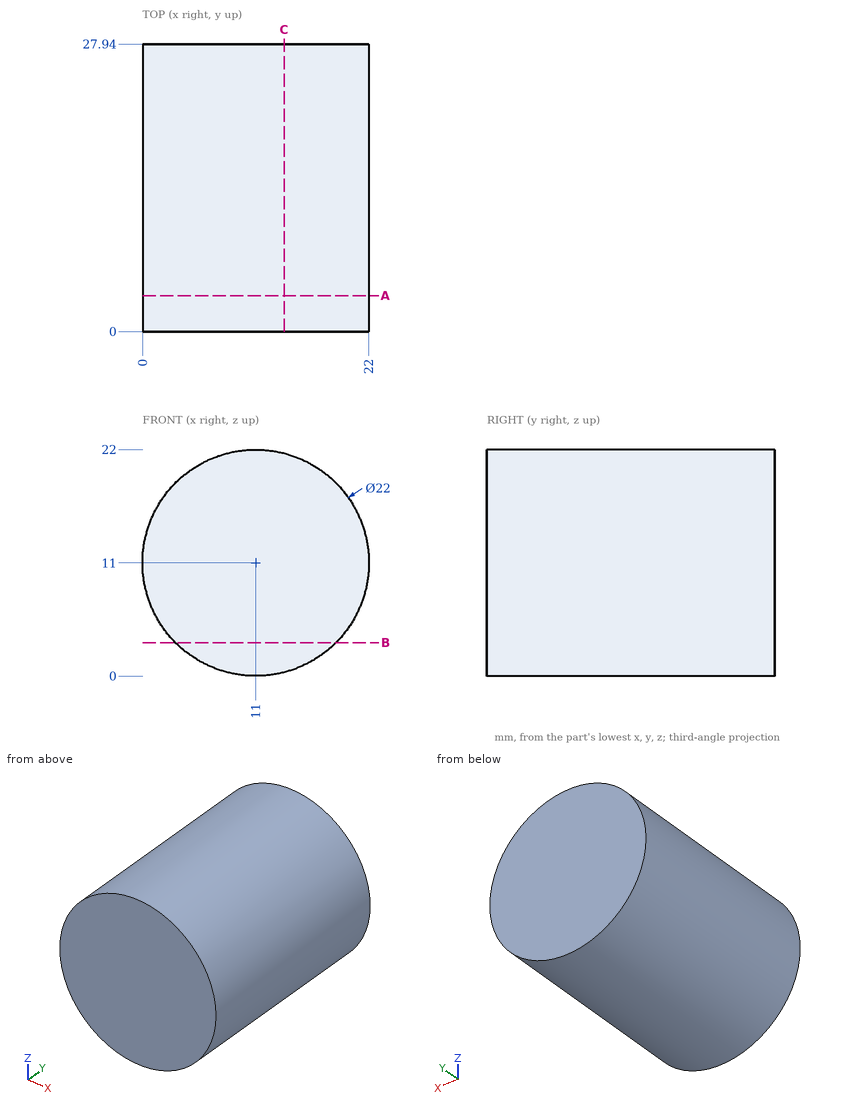
Geometry check sheet. Reference: drawing and pictorial views, mm from the part's lowest x, y, z. Give positions to 0.01 mm unless a question says otherwise; leave off trailing zeros. Order: outer loops, then holes, each group sorted by start corner. A loop starts at its lowest first (then second) coordinate and runs counter-clockwise, first axis right, second up. Notation, with made-up numbers: (-29.5, 74.25) -> (5.5, 74.25) arc R23 ccw to (5.5, 103.25) -> close; hole circle Ø1 at (71.5, 7). An arc over 180 degrees is marked (long way). Write each question's results on one line, items separated by ' | '. Start each with the question number.
(1) Gauge pin test, flat end, axial feed: P1, Ø8, axis at y = 13, z = 4.5, coming from the +X side. Record the tip position at first contact, or that the pin passes through.
(2) Sectioned sample at B-B (z = 3.25). Enter the section's corners in (x, y).
(3) Sectioned sample at A-A (y = 3.5). Enter the section's corners in (x, z), plus the area to 3 significant figures.
(4) Scan lines: line 1 (Z direction, x = 10.75, y = 21.25); line 2 (Z direction, x = 3.5, y = 11); line 3 (X direction, y = 26, z = 6.75). Record each from-to range of solid material in increasing order.
(5) Sectioned sample at C-C (x = 13.75). Enter the section's corners in (y, z), plus the area to 3 significant figures.
Answer below:
1) P1: x = 21.71
2) outline: (3.19, 0) -> (18.81, 0) -> (18.81, 27.94) -> (3.19, 27.94) -> close
3) outline: circle Ø22 at (11, 11) | area: 380 mm2
4) line 1: 0 to 22 | line 2: 2.95 to 19.05 | line 3: 0.85 to 21.15
5) outline: (0, 0.35) -> (27.94, 0.35) -> (27.94, 21.65) -> (0, 21.65) -> close | area: 595 mm2
